```python
from build123d import *

# Parameters (mm, degrees)
F0_R     = 17.78
F1_DEPTH = 25.4
F4_R     = 17.78
F4_R_2   = 16.8
F5_DEPTH = 10


with BuildPart() as f1:
    # F0 (on Front) → F1 (new body)
    with BuildSketch(Plane.XZ):
        Circle(F0_R)
    extrude(amount=F1_DEPTH)

    # F2 (on Top) → F3 (revolve, cut)
    with BuildSketch(Plane.XY):
        Polygon((0, -25.4), (0, 0), (-16.8, 0), (-1.3125, -25.4), align=None)
    revolve(axis=Axis((0, -12.7, 0), (0, -1, 0)), mode=Mode.SUBTRACT)

    # F4 (on face) → F5 (join)
    with BuildSketch(Plane(origin=(0, 0, 0), x_dir=(-1, 0, 0), z_dir=(0, 1, 0))):
        Circle(F4_R)
        Circle(F4_R_2, mode=Mode.SUBTRACT)
    extrude(amount=F5_DEPTH)


solid = f1.part
```
Here's how the part is built. I have some questions about the finished solid (model axes, mm). A direction names the side the tool comes from. Coordinates: 2 decimals unless noted, no trailing zeros. Order: outer loops, then holes, each group sorted by start corner. A loop starts at its lowest first (then second) coordinate and runs counter-clockwise, first axis right, second up. Notation, with made-up numbers: M 58.25,55.25 L 71.25,55.25 A28 cw 71.25,87.25 Z; hole C 71,-20 d2. An arc over 180 degrees is marked long. Answer as a JSON object with one key per item and string values. Group by question number.
(1) Suppose I cut it at C-C, the plane y = -15.5. Please give me the cut outline in (x, z), then the cut area to 3 significant figures.
(2) If we mould it in two halves opening along X, with no side actions, what happens to faces 3 (the face through (0, -25.4, -4)), 4 (the face through (1.567, -15.7, 7.055))? For each: released by +X, released by -X, zero draft, split by the parting line, or undercut.
(3) I need wall thicknesses on probe 1 along Z at (x, y) = (0, 7); probe 2 along X at (y, z) = (3, 10). Which ranges of each line are inside material? Lowest first, please.
(4) For pin 1 (2 mm diameter, centred on x = 4.5, y = -2.5, fed in from +Z); pin 2 (4 mm diameter, centred on x = 13.5, y = -14, fed in from -Z); pin 3 (5 mm diameter, centred on y = 2.5, z = -6.5, fed in from -X), each with a flat end and sliding along its axis, tell me the tip position at first contact or that it passes through.
(5) Which directions (+Z, -Z, +X, -X, +Y, -Y) give clear straight access to the entire face, cutting with the end or side of a thin tool? Please do faces 1 (the face through (-13, 10, 11)), 2 (the face through (-16.024, 4.93, 5.046)).
(6) Suppose I cut it at A-A, the plane z = 0. Please give me the cut outline in (x, y).
(7) Suppose I cut it at B-B, the plane x = 0. Please give me the cut outline in (y, z), then the cut area to 3 significant figures.
Values found:
{
 "1": {"outline": "C 0,0 d35.56; hole C 0,0 d14.7", "area": "823 mm^2"},
 "2": {"face 3": "zero draft", "face 4": "undercut"},
 "3": {"probe 1": "z = -17.78 to -16.8, 16.8 to 17.78", "probe 2": "x = -14.7 to -13.5, 13.5 to 14.7"},
 "4": {"pin 1": "stops at z = 17.43", "pin 2": "stops at z = -13.56", "pin 3": "stops at x = -17.32"},
 "5": {"face 1": "+Z, -Z, +X, -X, +Y", "face 2": "+Y"},
 "6": {"outline": "M -17.78,-25.4 L -1.31,-25.4 L -16.8,0 L -16.8,10 L -17.78,10 Z; M 1.31,-25.4 L 17.78,-25.4 L 17.78,10 L 16.8,10 L 16.8,0 Z"},
 "7": {"outline": "M -25.4,-17.78 L 10,-17.78 L 10,-16.8 L 0,-16.8 L -25.4,-1.31 Z; M -25.4,1.31 L 0,16.8 L 10,16.8 L 10,17.78 L -25.4,17.78 Z", "area": "463 mm^2"}
}
